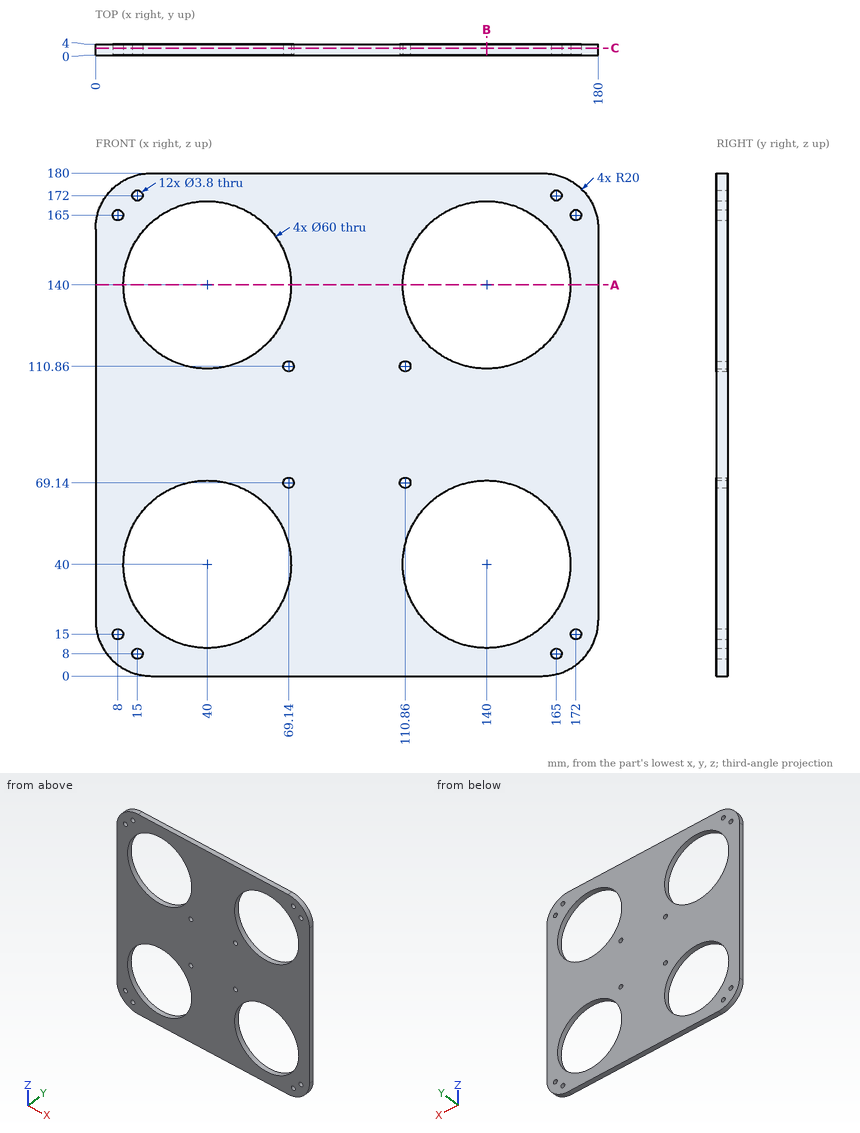
Check sheet for the drawn part. Datum: minimum x, y, z corner. Units: mm. Coordinates: 2 decimals unless noted, no trailing zeros. Order: outer loops, then holes, each group sorted by start corner. A loop starts at its lowest first (then second) coordinate and runs counter-clockwise, first axis right, second up. Notation, with made-up numbers: M -5.5,-35.75 L 27.5,-35.75 A16 cw 27.5,-8.75 Z; hole C 10.5,17.25 d4. An arc over 180 degrees is marked long. One line per item, written item: value. Start each with the question number.
Item 1: Scan lines: probe 1 along X at (y, z) = (2.35, 140); probe 2 along Z at (x, y) = (172, 1.65); probe 3 along Z at (x, y) = (165.5, 3.65) (1 decimal). Record each from-to range of solid material in increasing order.
Item 2: Sectioned sample at B-B (x = 140). Enter the section's corners in (y, z).
Item 3: Sectioned sample at A-A (z = 140). Enter the section's corners in (x, y), then the cut area to 3 significant figures.
Item 4: Sectioned sample at C-C (y = 2.55). Count the separate pieces of the cut face and the enclosed holes in it, then the cut area to 3 significant figures.
Conclusion:
1. probe 1: x = 0 to 10, 70 to 110, 170 to 180
1. probe 2: z = 4 to 13.1, 16.9 to 163.1, 166.9 to 176
1. probe 3: z = 0.8 to 6.2, 9.8 to 24.2, 55.8 to 124.2, 155.8 to 170.2, 173.8 to 179.2
2. outline: M 0,0 L 4,0 L 4,10 L 0,10 Z; M 0,70 L 4,70 L 4,110 L 0,110 Z; M 0,170 L 4,170 L 4,180 L 0,180 Z
3. outline: M 0,0 L 10,0 L 10,4 L 0,4 Z; M 70,0 L 110,0 L 110,4 L 70,4 Z; M 170,0 L 180,0 L 180,4 L 170,4 Z
3. area: 240 mm^2
4. separate pieces: 1
4. enclosed holes: 16
4. area: 20,600 mm^2
